The listing builds one solid part. Answer for the finished solid, in the listing's coordinates (mm). Round coordinates to 2 decimals unless told otherwise and drop trailing zeros. Write each loop counter-clockwise with the first axis right and the second up, starting at its lowest first coordinate (ties: lowest second). Pieces come first, ordered by that corner, then holes. Notation, with made-up numbers: (-36.5, -36.75) - (14.5, -36.75) arc R35 ccw to (14.5, -2.75) - close; hole circle Ø10 at (3.25, 46). An arc over 180 degrees is marked (long way). Use a Markdown table: item, result. Add a question column.
1) Find the intervals of material crossed by probe 1 along Y at (x, z) = (-15.75, 6); probe 2 along Y at (x, z) = (-10.5, -6.25); probe 3 along X at (y, z) = (-0.25, -5.5), in increasing order. Write a range as from..to.
2) Each of these flat-tipped pins is pushed along its axis until it touches: P1, Ø5, axis at x = -9, y = 11.5, coming from the +Z side; P2, Ø1, axis at x = -7, z = 1.5, coming from the -Y side; P3, Ø8, axis at x = -8, z = 1.5, coming from the -Y side; P4, Ø4, axis at x = -9.5, z = 5.5, coming from the +Y side. Where does it stop, or does it pass through?
3) A cutting plane is placed at A-A (x = -3). Give the vertices of the cut face in (y, z).
```python
from build123d import *

# Parameters (mm, degrees)
CROQUIS_BASE_DEPTH             = 6.9937
LENTE_PPAL_1_REACH             = 29.176
LENTE_PPAL_1_DIRECTION_2_REACH = 29.176
LENTE_PPAL_2_DEPTH             = 28.175928622
LENTE_PPAL_2_DEPTH_BACK        = 28.175928622
CROQUIS9_3_OUTSIDE_W           = 30.065
CROQUIS9_3_OUTSIDE_H           = 25.937
LENTE_START                    = -6.9937
LENTE_FRONTAL_DEPTH            = 13.9874
LENTE_TRASERA_DEPTH            = 13.9874


with BuildPart() as part:
    # Croquis1 → croquis base (new, symmetric)
    with BuildSketch(Plane.XY):
        with BuildLine():
            Line((-8.981845695, 12.608155172), (-23.035921146, 11.871612288))
            Line((-23.035921146, 11.871612288), (-23.035921146, 11.54013782))
            ThreePointArc((-23.035921146, 11.54013782), (-20.949684518, 9.582335705), (-18.945192114, 7.540918896))
            add(Edge.make_bspline(
                [(-18.945192114, 7.540918896), (-10.215008384, -3.697644103), (-2.846604825, -5.059081104)],
                knots=[0.497667241, 0.497667241, 0.497667241, 0.49955428, 0.49955428, 0.49955428], degree=2, weights=[1, 1, 1]))
            add(Edge.make_bspline(
                [(-2.846604825, -5.059081104), (-2.498165198, -4.87297933), (-2.177330418, -4.684462446)],
                knots=[0.498812075, 0.498812075, 0.498812075, 0.498911556, 0.498911556, 0.498911556], degree=2, weights=[1, 1, 1]))
            Line((-2.177330418, -4.684462446), (-2.177330418, 6.186438919))
            add(Edge.make_bspline(
                [(-2.177330418, 6.186438919), (-4.063319702, 8.141636997), (-6.994875026, 10.477389992)],
                knots=[0.50138293, 0.50138293, 0.50138293, 0.502013312, 0.502013312, 0.502013312], degree=2, weights=[1, 1, 1]))
            Line((-6.994875026, 10.477389992), (-8.981845695, 12.608155172))
        make_face()
    extrude(amount=CROQUIS_BASE_DEPTH, both=True)

    # lente ppal 1: up to this face of the body (flat: up to its plane)
    lente_ppal_1_end = Plane(part.part.faces().sort_by_distance((-10.153546236, 5.159655325, 6.9937))[0])
    # Croquis9 → lente ppal 1 (add, up to the picked face)
    with BuildSketch(Plane.XY, mode=Mode.PRIVATE) as lente_ppal_1_sk1:
        with BuildLine():
            add(Edge.make_bspline(
                [(-2.177330418, -4.388282022), (-10.4130765, -4.994158739), (-19.969359014, 9.493765032)],
                knots=[0, 0, 0, 1, 1, 1], degree=2))
            Line((-19.969359014, 9.493765032), (-10.309820395, 10))
            Line((-10.309820395, 10), (-2.177330418, 6.082860828))
            Line((-2.177330418, 6.082860828), (-2.177330418, 2.424232079))
            add(Edge.make_bspline(
                [(-2.177330418, 2.424232079), (-0.304369248, 0.128042884), (-2.177330418, -1.840420572)],
                knots=[0, 0, 0, 1, 1, 1], degree=2))
            Line((-2.177330418, -1.840420572), (-2.177330418, -4.388282022))
        make_face()
    lente_ppal_1_tool1 = split(extrude(lente_ppal_1_sk1.sketch, amount=LENTE_PPAL_1_REACH, mode=Mode.PRIVATE), bisect_by=lente_ppal_1_end, keep=Keep.BOTH, mode=Mode.PRIVATE)
    add(lente_ppal_1_tool1.solids().sort_by(Axis((-9.106368, 3.599172, 0), (0, 0, 1)))[0])

    # lente ppal 1 direction 2: up to this face of the body (flat: up to its plane)
    lente_ppal_1_direction_2_end = Plane(part.part.faces().sort_by_distance((-10.153546236, 5.159655325, -6.9937))[0])
    # Croquis9 → lente ppal 1 direction 2 (add, up to the picked face)
    with BuildSketch(Plane.XY, mode=Mode.PRIVATE) as lente_ppal_1_direction_2_sk1:
        with BuildLine():
            add(Edge.make_bspline(
                [(-2.177330418, -4.388282022), (-10.4130765, -4.994158739), (-19.969359014, 9.493765032)],
                knots=[0, 0, 0, 1, 1, 1], degree=2))
            Line((-19.969359014, 9.493765032), (-10.309820395, 10))
            Line((-10.309820395, 10), (-2.177330418, 6.082860828))
            Line((-2.177330418, 6.082860828), (-2.177330418, 2.424232079))
            add(Edge.make_bspline(
                [(-2.177330418, 2.424232079), (-0.304369248, 0.128042884), (-2.177330418, -1.840420572)],
                knots=[0, 0, 0, 1, 1, 1], degree=2))
            Line((-2.177330418, -1.840420572), (-2.177330418, -4.388282022))
        make_face()
    lente_ppal_1_direction_2_tool1 = split(extrude(lente_ppal_1_direction_2_sk1.sketch, amount=-LENTE_PPAL_1_DIRECTION_2_REACH, mode=Mode.PRIVATE), bisect_by=lente_ppal_1_direction_2_end, keep=Keep.BOTH, mode=Mode.PRIVATE)
    add(lente_ppal_1_direction_2_tool1.solids().sort_by(Axis((-9.106368, 3.599172, 0), (0, 0, -1)))[0])

    # Croquis9_3 outside → lente ppal 2 (cut, two sides: drawn at the far end of the back side and taken through both)
    with BuildSketch(Plane.XY.offset(-LENTE_PPAL_2_DEPTH_BACK)):
        with Locations((-12.1385, 3.7745)):
            Rectangle(CROQUIS9_3_OUTSIDE_W, CROQUIS9_3_OUTSIDE_H)
        with BuildLine():
            Line((-2.177330418, -1.840420572), (-2.177330418, -4.388282022))
            add(Edge.make_bspline(
                [(-2.177330418, -4.388282022), (-10.4130765, -4.994158739), (-19.969359014, 9.493765032)],
                knots=[0, 0, 0, 1, 1, 1], degree=2))
            Line((-19.969359014, 9.493765032), (-10.309820395, 10))
            Line((-10.309820395, 10), (-2.177330418, 6.082860828))
            Line((-2.177330418, 6.082860828), (-2.177330418, 2.424232079))
            add(Edge.make_bspline(
                [(-2.177330418, 2.424232079), (-0.304369248, 0.128042884), (-2.177330418, -1.840420572)],
                knots=[0, 0, 0, 1, 1, 1], degree=2))
        make_face(mode=Mode.SUBTRACT)
    extrude(amount=LENTE_PPAL_2_DEPTH + LENTE_PPAL_2_DEPTH_BACK, mode=Mode.SUBTRACT)

    # Croquis8 → lente frontal (add)
    with BuildSketch(Plane.XY.offset(LENTE_START)):
        with BuildLine():
            Line((0.1, 2.877673418), (0.1, 15.587903347))
            Line((0.1, 15.587903347), (-1.059110992, 15.277320493))
            Line((-1.059110992, 15.277320493), (-2.200378811, 14.9065001))
            Line((-2.200378811, 14.9065001), (-3.324385438, 14.486251242))
            Line((-3.324385438, 14.486251242), (-4.38392255, 13.922885367))
            Line((-4.38392255, 13.922885367), (-5.329535454, 13.184091597))
            Line((-5.329535454, 13.184091597), (-6.132492182, 12.292317806))
            Line((-6.132492182, 12.292317806), (-6.768395299, 11.274660091))
            Line((-6.768395299, 11.274660091), (-7.217923211, 10.162039465))
            Line((-7.217923211, 10.162039465), (-10.309820395, 10))
            Line((-10.309820395, 10), (-2.177330418, 2.342487007))
            Line((-2.177330418, 2.342487007), (-1.190501641, 2.376947827))
            add(Edge.make_bspline(
                [(-1.190501641, 2.376947827), (-0.463368169, 2.402339888), (0.1, 2.877673418)],
                knots=[0, 0, 0, 1, 1, 1], degree=2))
        make_face()
    extrude(amount=LENTE_FRONTAL_DEPTH)

    # Croquis11 → lente trasera (add)
    with BuildSketch(Plane.XY.offset(LENTE_START)):
        with BuildLine():
            Line((0.1, -2.960353775), (0.1, -3.460353775))
            Line((0.1, -3.460353775), (-3.810712242, -6))
            Line((-3.810712242, -6), (-9.112438619, -1.551323352))
            Line((-9.112438619, -1.551323352), (-1.965100505, -1.800913899))
            add(Edge.make_bspline(
                [(-1.965100505, -1.800913899), (-0.923066369, -1.837302533), (0.1, -2.960353775)],
                knots=[0, 0, 0, 1, 1, 1], degree=2))
        make_face()
    extrude(amount=LENTE_TRASERA_DEPTH)


solid = part.part
```
Entries:
| question | item | result |
|---|---|---|
| 1 | probe 1 | y = 3.76..9.71 |
| 1 | probe 2 | y = -1.41..9.99 |
| 1 | probe 3 | x = -11.91..-1.29 |
| 2 | P1 | stops at z = 6.99 |
| 2 | P2 | stops at y = -3.74 |
| 2 | P3 | stops at y = -5.84 |
| 2 | P4 | stops at y = 10.15 |
| 3 | outline | (-5.47, -6.99) - (14.61, -6.99) - (14.61, 6.99) - (-5.47, 6.99) - close |
